For this review, use the dimensioned drawing (mm, ordinates from the lowest corner) and the shaded views. Give positions to 0.01 mm unless a question says otherwise; leave off trailing zeros. Order: outer loops, then holes, each group sorted by start corner. A loop starts at its lowest first (then second) coordinate and runs counter-clockwise, first axis right, second up. Notation, with made-up numbers: M -35.5,75 L 21.5,75 A23 cw 21.5,113 Z; hole C 37,52.25 d3. An arc over 180 degrees is marked long. Use CSV: the item, a comma, the result in double quotes. Start each with the question number.
(1) Draft analysis for pull direction Z (two halves, no side actions). For the marked faces 1, 2 and 3, state which applies: pulls with the +Z half, pulls with the -Z half, needs draft (parallel to the pull), parting line crosses it, or undercut.
(2) Consider section C-C (x = 46). Write out the cut boundary in (y, z), and give its area (3 significant figures).
(3) Consider section D-D (z = 44.5). Write out the cut boundary in (x, y).
(4) Consider section B-B (z = 34). Write out the cut boundary in (x, y).
(5) Wall thickness on L1, parallel to X at y = 33, z = 25; L2, parallel to Z at x = 50, y = 33; L3, parallel to X at y = 3.5, z = 37: over which ranges is each line inside the solid? List them lowest first. Write a range as from..to.
(6) Consider section A-A (y = 18.5). Write out the cut boundary in (x, z), and give its area (3 significant figures).
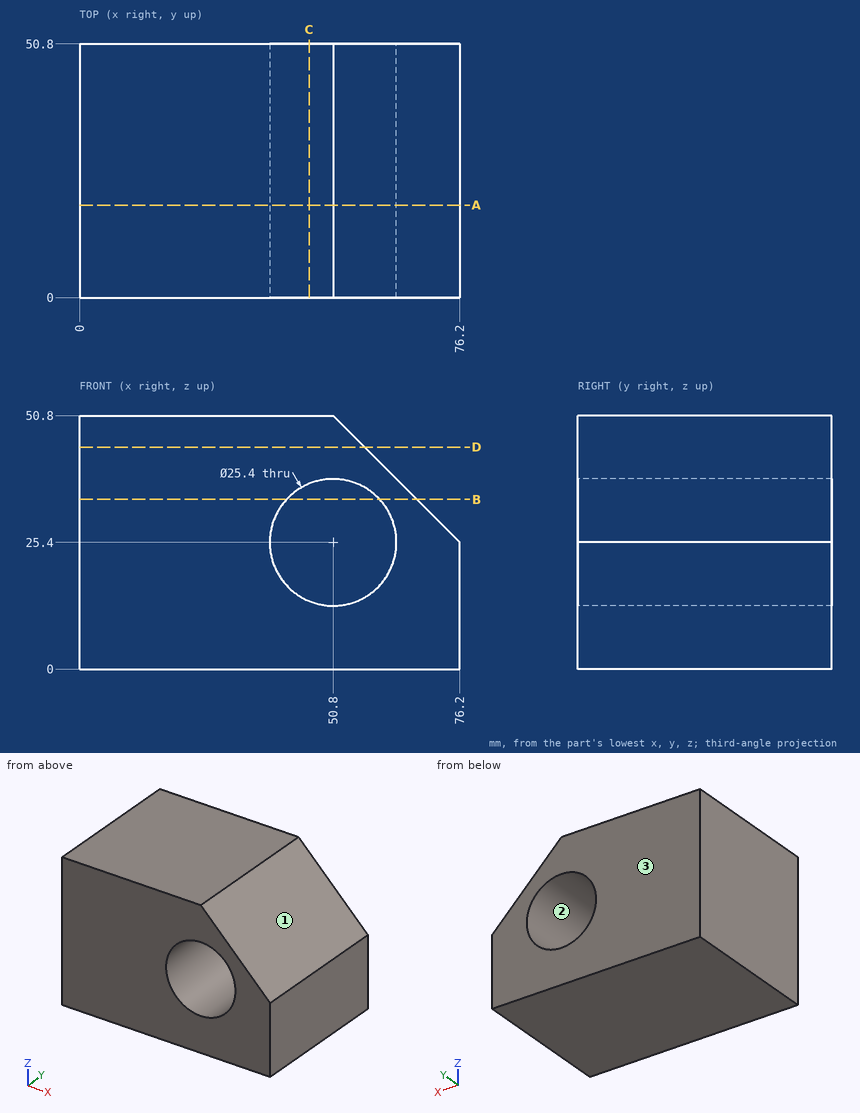
Check result:
1,face 1,"pulls with the +Z half"
1,face 2,"undercut"
1,face 3,"needs draft"
2,outline,"M 0,0 L 50.8,0 L 50.8,13.64 L 0,13.64 Z; M 0,37.16 L 50.8,37.16 L 50.8,50.8 L 0,50.8 Z"
2,area,"1,390 mm^2"
3,outline,"M 0,0 L 57.1,0 L 57.1,50.8 L 0,50.8 Z"
4,outline,"M 0,0 L 41.45,0 L 41.45,50.8 L 0,50.8 Z; M 60.15,0 L 67.6,0 L 67.6,50.8 L 60.15,50.8 Z"
5,L1,"x = 0..38.11, 63.49..76.2"
5,L2,"z = 0..12.73, 38.07..50.8"
5,L3,"x = 0..45.63, 55.97..64.6"
6,outline,"M 0,0 L 76.2,0 L 76.2,25.4 L 50.8,50.8 L 0,50.8 Z; hole C 50.8,25.4 d25.4"
6,area,"3,040 mm^2"
